Answer from the drawing. Dimensions are ordinates in mm from the lowest x, y and z of the part. Coordinates: 2 decimals unless noted, no trailing zeros. Order: outer loops, then holes, each group sorted by start corner. A loop starts at its lowest first (then second) coordinate and runs counter-clockwise, first axis right, second up.
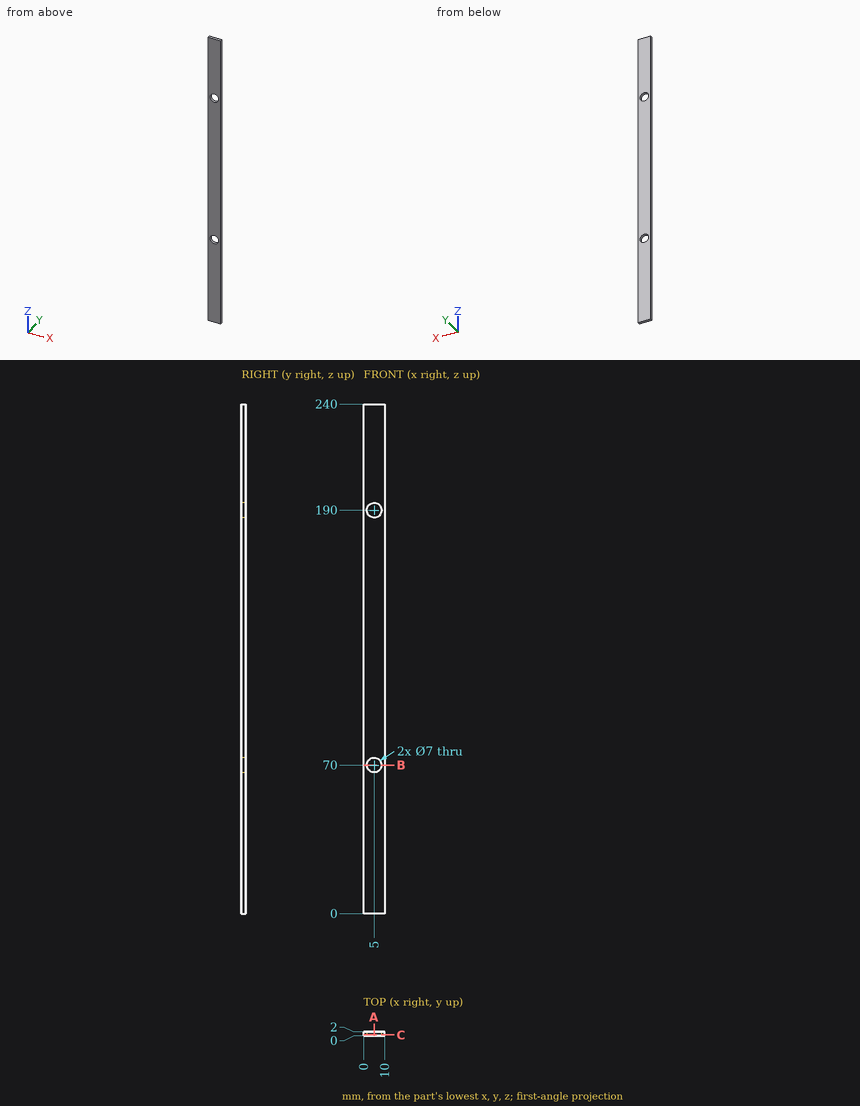
1) Section C-C (y = 0.5) is taken. Give the vertices of the cut face in (x, z).
2) Section B-B (z = 70) is taken. Give the vertices of the cut face in (x, y), then the cut area to 3 significant figures.
3) Each of these flat-tipped pins is pushed along its axis until it touches: P1, Ø4, axis at x = 7, z = 195, coming from the -Y side; P2, Ø4, axis at x = 5, z = 70, coming from the -Y side. Where does it stop, or does it pass through?
4) Section A-A (x = 5) is taken. Give the vertices of the cut face in (y, z).
5) Consider L1, parallel to Z at x = 5, y = 1.25; L2, parallel to Z at x = 2, y = 0.35; L3, parallel to X at y = 1.3, z = 190. Determine where each line is inside the solid, lowest interval first.
Filled sheet:
1. outline: (0, 0) - (10, 0) - (10, 240) - (0, 240) - close; hole circle Ø7 at (5, 70); hole circle Ø7 at (5, 190)
2. outline: (0, 0) - (1.5, 0) - (1.5, 2) - (0, 2) - close; (8.5, 0) - (10, 0) - (10, 2) - (8.5, 2) - close
2. area: 6.00 mm2
3. P1: stops at y = 0
3. P2: passes through
4. outline: (0, 0) - (2, 0) - (2, 66.5) - (0, 66.5) - close; (0, 73.5) - (2, 73.5) - (2, 186.5) - (0, 186.5) - close; (0, 193.5) - (2, 193.5) - (2, 240) - (0, 240) - close
5. L1: z = 0 to 66.5, 73.5 to 186.5, 193.5 to 240
5. L2: z = 0 to 68.2, 71.8 to 188.2, 191.8 to 240
5. L3: x = 0 to 1.5, 8.5 to 10
